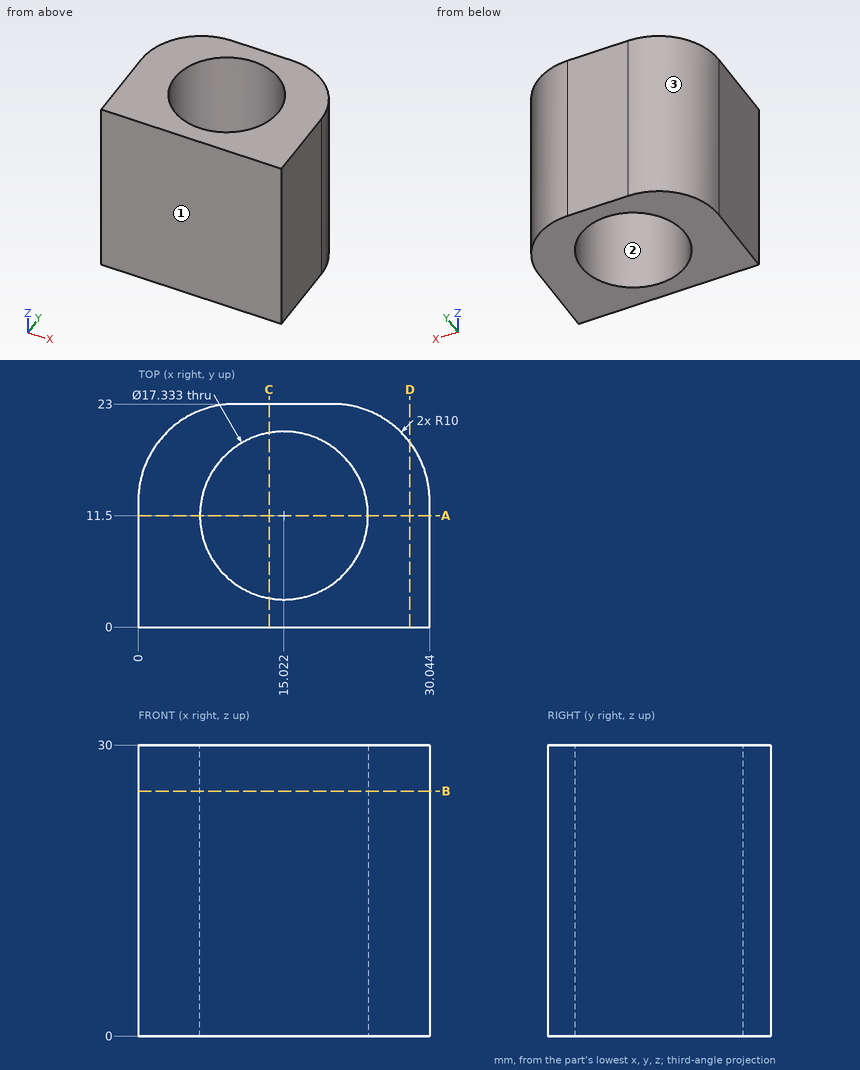
Source: three-view drawing plus pictorial views. Frame: mm from the lowest corner of the part. Give positions to 0.01 mm unless a question says otherwise; leave off trailing zeros. Write each loop counter-clockwise with the first axis right and the second up, starting at its lowest first coordinate (ties: lowest second). Pieces come first, ordered by that corner, then holes. Notation, with made-up numbers: (0, -17) - (38, -17) arc R4 ccw to (38, -10) - close; hole circle Ø5 at (64.25, 77.25). An arc over 180 degrees is marked (long way). Write item = value, one per line. Start each with the question number.
Q1. Cut plane C-C, the plane x = 13.5. Return loops of the section in (y, z), then the cut area to 3 significant figures.
Q2. Cut plane D-D, the plane x = 28. Return loops of the section in (y, z), then the cut area to 3 significant figures.
Q3. Cut plane A-A, the plane y = 11.5. Return loops of the section in (x, z) (1 decimal), then the cut area to 3 significant figures.
Q4. Pin query (flat end, axial travel): pin 1 Ø1.5 at (y, z) = (15.5, 15) entering from -X (1 decimal). Return the tip coordinate at first contact, or that it passes through.
Q5. Cut plane B-B, the plane z = 25.25. Return loops of the section in (x, y), then the cut area to 3 significant figures.
Q6. Draft query along Y for the marked faces 1, 2 and 3. Return one class per face: +Y half, -Y half, draft (parallel to the pull), parting line (faces both ways), or undercut.
Q7. Material intervals for probe 1 along Y at (x, z) = (21, 20) (1 decimal); probe 2 along X at (y, z) = (6.5, 14.5) (1 decimal); probe 3 along X at (y, z) = (14.5, 8), sorted ascending.
Computed values:
q1.outline = (0, 0) - (2.97, 0) - (2.97, 30) - (0, 30) - close; (20.03, 0) - (23, 0) - (23, 30) - (20.03, 30) - close
q1.area = 178 mm²
q2.outline = (0, 0) - (19.06, 0) - (19.06, 30) - (0, 30) - close
q2.area = 572 mm²
q3.outline = (0, 0) - (6.4, 0) - (6.4, 30) - (0, 30) - close; (23.7, 0) - (30, 0) - (30, 30) - (23.7, 30) - close
q3.area = 381 mm²
q4.pin_1 = 0.2
q5.outline = (0, 0) - (30.04, 0) - (30.04, 13) arc R10 ccw to (20.04, 23) - (10, 23) arc R10 ccw to (0, 13) - close; hole circle Ø17.33 at (15.02, 11.5)
q5.area = 412 mm²
q6.face_1 = -Y half
q6.face_2 = undercut
q6.face_3 = +Y half
q7.probe_1 = 0 to 5.2, 17.8 to 23
q7.probe_2 = 0 to 7.9, 22.1 to 30
q7.probe_3 = 0.11 to 6.89, 23.15 to 29.93
